Can you work these out from the model? Positions are in its coordinate system, mm. Face numbers are marked on the shaded views. Coordinates: 2 decimals unless noted, no trailing zeros. Write each loop counter-clockwise with the first axis right and the second up, starting at its lowest first coordinate (ties: lowest second). Pieces come first, ordered by that corner, then holes. Notation, with made-up numbers: M 42,68.25 L 84,68.25 A15 ccw 84,81.25 Z; hole C 1.25,12 d10. An arc over 180 degrees is marked long. Use one line per item in the form item = value. Start each with the question number.
```python
from build123d import *

# Parameters (mm, degrees)
F0_R     = 4
F1_DEPTH = 5
F2_R     = 1
F3_R     = 2.25
F4_DEPTH = 3


with BuildPart() as f1:
    # F0 (on Top) → F1 (new body)
    with BuildSketch(Plane.XY):
        Circle(F0_R)
    extrude(amount=F1_DEPTH)

    # F2
    f2_edges = [f1.edges().sort_by_distance(p)[0] for p in [
        (-4, 0, 5),
    ]]
    fillet(f2_edges, radius=F2_R)

    # F3 (on face) → F4 (cut)
    with BuildSketch(Plane(origin=(0, 0, 0), x_dir=(1, 0, 0), z_dir=(0, 0, -1))):
        Circle(F3_R)
    extrude(amount=-F4_DEPTH, mode=Mode.SUBTRACT)


solid = f1.part
```
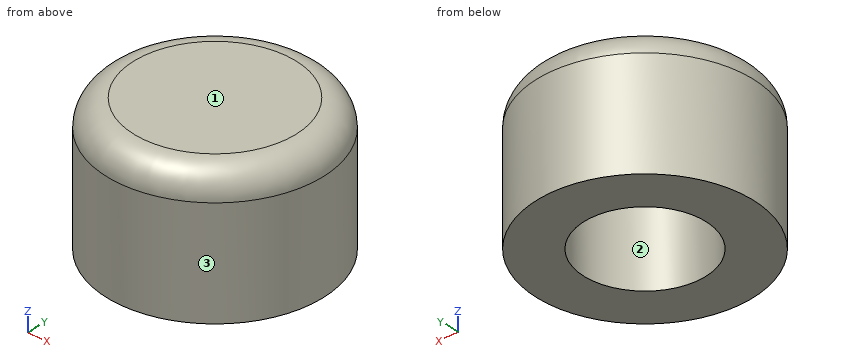
1) If we mould it in two halves opening along Y, with no side actions, what happens to the marked faces 1, 2 and 3? For each: +Y half, -Y half, draft (parallel to the pull), parting line (faces both ways), or undercut.
2) Please list where these lines run through material, in increasing order: line 1 (Y direction, x = 0, z = 0.7); line 2 (Z direction, x = -0.75, y = -0.5); line 3 (X direction, y = -1, z = 0.55).
3) Suppose I cut it at C-C on z = 1.3. Please give me the cut outline in (x, y), and give its area (3 significant figures).
4) Suppose I cut it at A-A on y = 0. Please give me the cut outline in (x, z), and give its area (3 significant figures).
Computed values:
q1.face_1 = draft
q1.face_2 = undercut
q1.face_3 = parting line
q2.line_1 = -4 to -2.25, 2.25 to 4
q2.line_2 = 3 to 5
q2.line_3 = -3.87 to -2.02, 2.02 to 3.87
q3.outline = C 0,0 d8; hole C 0,0 d4.5
q3.area = 34.4 mm²
q4.outline = M -4,0 L -2.25,0 L -2.25,3 L 2.25,3 L 2.25,0 L 4,0 L 4,4 A1 ccw 3,5 L -3,5 A1 ccw -4,4 Z
q4.area = 26.1 mm²
